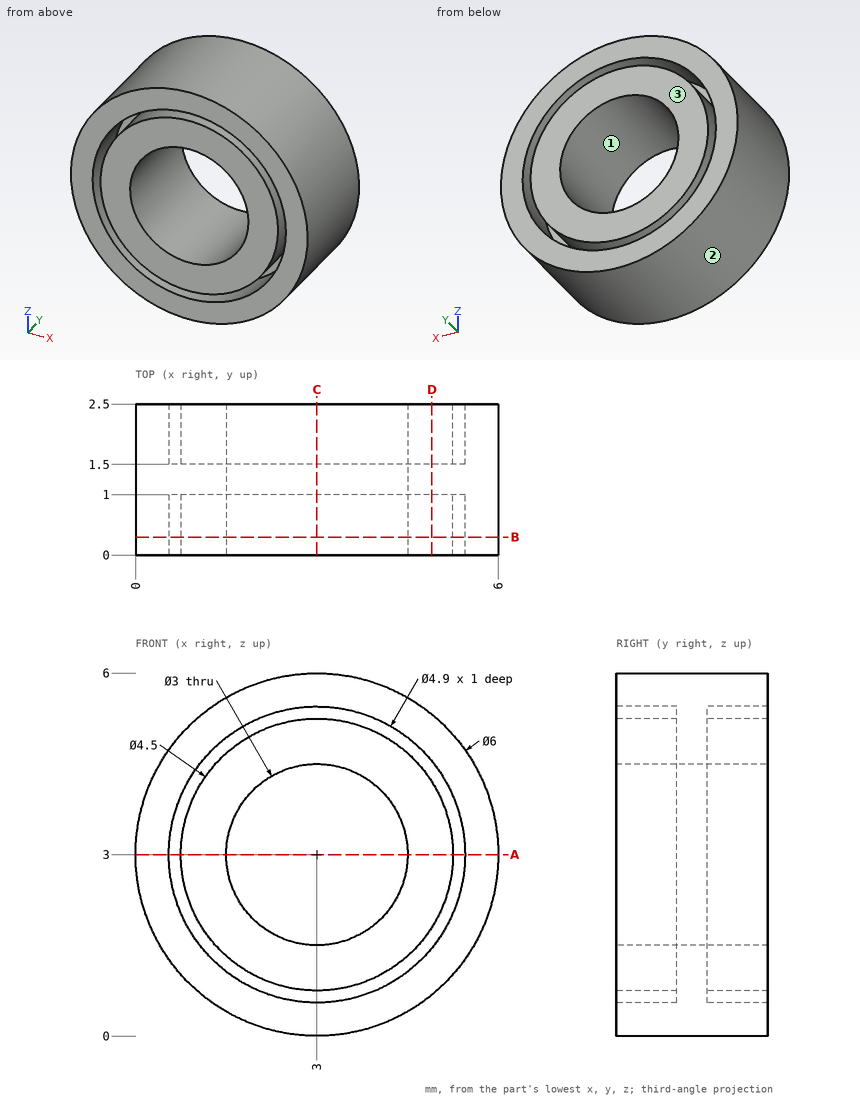
Design review of the part shown in the three views and the two pictorial views. Dimensions are in mm from the part's minimum x, y and z. Give positions to 0.01 mm unless a question says otherwise; leave off trailing zeros. Loops run counter-clockwise (first coordinate to the right, second up) from the corner with the lowest first, then second, coordinate; pieces in that order, holes last. Notation, with made-up numbers: (78.5, -37.75) -> (109.5, -37.75) arc R25 cw to (109.5, 0.25) -> close; hole circle Ø4 at (38, 20.5). An arc over 180 degrees is marked (long way). Answer as a JSON object with one key per item and string values. Group by question number.
Q1. Take a section at A-A (z = 3). Write out the cut boundary in (x, y), plus the area to 3 significant figures.
Q2. Take a section at C-C (x = 3). Write out the cut boundary in (y, z).
Q3. Insertion check: pin 1 (1 mm diameter, centred on y = 0.5, z = 2, fed in from +X). The pin has a flat end and moves straight along its axis. Give the tip position at first contact, or say it passes through.
Q4. Wall thickness on line 1 along X through (y, z) = (0.5, 3); line 2 along X through (y, z) = (0.5, 4.65); line 3 along Z through (x, y) = (3.65, 1.55): over which ranges is each line inside the solid? List them lowest first.
Q5. Draft analysis for pull direction X (two halves, no side actions). For the marked faces 1, 2 and 3, state which applies: pulls with the +X half, pulls with the -X half, needs draft (parallel to the pull), parting line crosses it, or undercut.
Q6. Take a section at B-B (y = 0.3). Write out the cut boundary in (x, z), plus the area to 3 significant figures.
Q7. Take a section at D-D (x = 4.9). Write out the cut boundary in (y, z).
Answer below:
{
 "1": {"outline": "(0, 0) -> (0.55, 0) -> (0.55, 1) -> (0.75, 1) -> (0.75, 0) -> (1.5, 0) -> (1.5, 2.5) -> (0.75, 2.5) -> (0.75, 1.5) -> (0.55, 1.5) -> (0.55, 2.5) -> (0, 2.5) -> close; (4.5, 0) -> (5.25, 0) -> (5.25, 1) -> (5.45, 1) -> (5.45, 0) -> (6, 0) -> (6, 2.5) -> (5.45, 2.5) -> (5.45, 1.5) -> (5.25, 1.5) -> (5.25, 2.5) -> (4.5, 2.5) -> close", "area": "6.70 mm2"},
 "2": {"outline": "(0, 0) -> (2.5, 0) -> (2.5, 0.55) -> (1.5, 0.55) -> (1.5, 0.75) -> (2.5, 0.75) -> (2.5, 1.5) -> (0, 1.5) -> (0, 0.75) -> (1, 0.75) -> (1, 0.55) -> (0, 0.55) -> close; (0, 4.5) -> (2.5, 4.5) -> (2.5, 5.25) -> (1.5, 5.25) -> (1.5, 5.45) -> (2.5, 5.45) -> (2.5, 6) -> (0, 6) -> (0, 5.45) -> (1, 5.45) -> (1, 5.25) -> (0, 5.25) -> close"},
 "3": {"pin 1": "stops at x = 5.96"},
 "4": {"line 1": "x = 0 to 0.55, 0.75 to 1.5, 4.5 to 5.25, 5.45 to 6", "line 2": "x = 0.49 to 1.19, 1.47 to 4.53, 4.81 to 5.51", "line 3": "z = 0.07 to 0.64, 0.85 to 1.65, 4.35 to 5.15, 5.36 to 5.93"},
 "5": {"face 1": "undercut", "face 2": "parting line crosses it", "face 3": "needs draft"},
 "6": {"outline": "circle Ø6 at (3, 3); circle Ø4.5 at (3, 3); hole circle Ø4.9 at (3, 3); hole circle Ø3 at (3, 3)", "area": "18.3 mm2"},
 "7": {"outline": "(0, 0.68) -> (2.5, 0.68) -> (2.5, 1.45) -> (1.5, 1.45) -> (1.5, 1.79) -> (2.5, 1.79) -> (2.5, 4.21) -> (1.5, 4.21) -> (1.5, 4.55) -> (2.5, 4.55) -> (2.5, 5.32) -> (0, 5.32) -> (0, 4.55) -> (1, 4.55) -> (1, 4.21) -> (0, 4.21) -> (0, 1.79) -> (1, 1.79) -> (1, 1.45) -> (0, 1.45) -> close"}
}
